```python
from build123d import *

# Parameters (mm, degrees)
F0_R     = 1
F2_DEPTH = 8
F0_R_2   = 2.667
F3_DEPTH = 27.5
F4_DEPTH = 31
F5_DEPTH = 23.5


with BuildPart() as f2:
    # F0 (on Top) → F2 (new body)
    with BuildSketch(Plane.XY):
        with BuildLine():
            Line((1.5, 24.5531070977), (0, 24.5531070977))
            Line((0, 24.5531070977), (-1.5, 24.5531070977))
            ThreePointArc((-1.5, 24.5531070977), (-5.7426406871, 26.3104664106), (-7.5, 30.5531070977))
            Line((-7.5, 30.5531070977), (-7.5, 8.1781070977))
            ThreePointArc((-7.5, 8.1781070977), (-6.9142135624, 6.7638935354), (-5.5, 6.1781070977))
            Line((-5.5, 6.1781070977), (5.5, 6.1781070977))
            ThreePointArc((5.5, 6.1781070977), (6.9142135624, 6.7638935354), (7.5, 8.1781070977))
            Line((7.5, 8.1781070977), (7.5, 30.5531070977))
            ThreePointArc((7.5, 30.5531070977), (5.7426406871, 26.3104664106), (1.5, 24.5531070977))
        make_face()
        with Locations((0, 11.1781070977)):
            Circle(F0_R, mode=Mode.SUBTRACT)
        with Locations((0, 20.6781070977)):
            Circle(F0_R, mode=Mode.SUBTRACT)
    extrude(amount=F2_DEPTH)

    # F0 (on Top) → F3 (join)
    with BuildSketch(Plane.XY):
        with BuildLine():
            Line((-1.5, 24.5531070977), (0, 24.5531070977))
            Line((0, 24.5531070977), (1.5, 24.5531070977))
            ThreePointArc((1.5, 24.5531070977), (5.7426406871, 26.3104664106), (7.5, 30.5531070977))
            Line((7.5, 30.5531070977), (7.5, 46.1781070977))
            ThreePointArc((7.5, 46.1781070977), (5.7426406871, 50.4207477849), (1.5, 52.1781070977))
            Line((1.5, 52.1781070977), (-1.5, 52.1781070977))
            ThreePointArc((-1.5, 52.1781070977), (-5.7426406871, 50.4207477849), (-7.5, 46.1781070977))
            Line((-7.5, 46.1781070977), (-7.5, 30.5531070977))
            ThreePointArc((-7.5, 30.5531070977), (-5.7426406871, 26.3104664106), (-1.5, 24.5531070977))
        make_face()
        with BuildLine():
            ThreePointArc((0, 24.5531070977), (-1.8561553006, 29.0342623984), (2.625, 27.1781070977))
            ThreePointArc((2.625, 27.1781070977), (1.8561553006, 25.3219517971), (0, 24.5531070977))
        make_face(mode=Mode.SUBTRACT)
        with Locations((0, 47.1781070977)):
            Circle(F0_R_2, mode=Mode.SUBTRACT)
        with BuildLine():
            ThreePointArc((0, 24.5531070977), (1.8561553006, 25.3219517971), (2.625, 27.1781070977))
            ThreePointArc((2.625, 27.1781070977), (-1.8561553006, 29.0342623984), (0, 24.5531070977))
        make_face()
    extrude(amount=F3_DEPTH)

    # F0 (on Top) → F4 (join)
    with BuildSketch(Plane.XY):
        with BuildLine():
            ThreePointArc((0, 24.5531070977), (1.8561553006, 25.3219517971), (2.625, 27.1781070977))
            ThreePointArc((2.625, 27.1781070977), (-1.8561553006, 29.0342623984), (0, 24.5531070977))
        make_face()
    extrude(amount=F4_DEPTH)

    # F0 (on Top) → F5 (join)
    with BuildSketch(Plane.XY):
        with Locations((0, 47.1781070977)):
            Circle(F0_R_2)
    extrude(amount=F5_DEPTH)


solid = f2.part
```
CAD build for the part. Positions are in the model's coordinates, mm. A direction names the side the tool comes from. Coordinates: 2 decimals unless noted, no trailing zeros. Order: outer loops, then holes, each group sorted by start corner. A loop starts at its lowest first (then second) coordinate and runs counter-clockwise, first axis right, second up. Notation, with made-up numbers: M -17.5,62 L 8.5,62 A26 cw 8.5,98 Z; hole C 70,46.5 d5. An arc over 180 degrees is marked long. Answer as CSV lines item,"result".
1) Mould opens along X. For faces 1 (the cylindrical face through (1.23, 44.81, 25.47)), 2 (the cylindrical face through (-6.93, 6.78, 3.94)), 3 (the flat face through (0, 24.553, 18)) say: released by +X, released by -X, zero draft, split by the parting line, or undercut.
Verdict:
face 1,"undercut"
face 2,"released by -X"
face 3,"zero draft"
2) Drill centre lines: L1, parallel to Y at x = 0, z = 1.5; L2, parallel to Y at x = 0, z = 25.85; L3, parallel to Y at x = 0.25, z = 10. Where is each one in solid material? Low to high. Write a range as from..to.
Verdict:
L1,"6.18..10.18, 12.18..19.68, 21.68..52.18"
L2,"24.55..44.51, 49.85..52.18"
L3,"24.55..52.18"
3) Cut at D-D (x = 4). List the corners of the cut face in (y, z).
Verdict:
outline,"M 6.18,0 L 51.63,0 L 51.63,27.5 L 25.1,27.5 L 25.1,8 L 6.18,8 Z"
4) Cut at B-B (z = 11). List the corners of the cut face in (x, y), then the cut area to 3 significant figures.
Verdict:
outline,"M -7.5,30.55 A6 ccw -1.5,24.55 L 1.5,24.55 A6 ccw 7.5,30.55 L 7.5,46.18 A6 ccw 1.5,52.18 L -1.5,52.18 A6 ccw -7.5,46.18 Z"
area,"383 mm2"
5) Flat gauge pins, fed straight in: P1, Ø2.5, axis at x = -0.5, z = 16.5, coming from the -Y side; P2, Ø5, axis at x = 0, y = 47.18, coming from the +Z side; P3, Ø4.5, axis at x = -3.5, y = 13.5, coming from the +Z side. Where does each tip first touch, or does it go through?
Verdict:
P1,"y = 24.55"
P2,"z = 23.5"
P3,"z = 8"
6) Cut at A-A (z = 3). List the corners of the cut face in (x, y).
Verdict:
outline,"M -7.5,8.18 A2 ccw -5.5,6.18 L 5.5,6.18 A2 ccw 7.5,8.18 L 7.5,46.18 A6 ccw 1.5,52.18 L -1.5,52.18 A6 ccw -7.5,46.18 Z; hole C 0,11.18 d2; hole C 0,20.68 d2"
7) 3-axis set-ups, long thin cutter, end or side, ignore diameter. For faces 4 (the cylindrical face through (-5.79, 26.36, 17.61)), 5 (the cylindrical face through (5.696, 26.264, 17.614)), 6 (the flat face through (0, 47, 23.5)), 7 (the flat face through (0, 30, 0)), 8 (the flat face through (0, 27, 31)): which of +Z, -Z, +X, -X, +Y, -Y reach the whole face in a straight line?
Verdict:
face 4,"+Z, -X, -Y"
face 5,"+Z, +X, -Y"
face 6,"+Z"
face 7,"-Z, +X, -X, +Y, -Y"
face 8,"+Z, +X, -X, +Y, -Y"
8) Cut at C-C (y = 33). List the corners of the cut face in (x, z).
Verdict:
outline,"M -7.5,0 L 7.5,0 L 7.5,27.5 L -7.5,27.5 Z"
